Read the model definition and answer for the solid it produces. Units are mm, in the model's axes. A direction names the side the tool comes from. Coordinates: 2 decimals unless noted, no trailing zeros. Loops run counter-clockwise (first coordinate to the right, second up) from the corner with the lowest first, then second, coordinate; pieces in that order, holes last. Notation, with made-up numbers: (20.25, 11.25) - (26.25, 11.25) arc R29 ccw to (26.25, 31.25) - close; hole circle Ø7 at (71.25, 69.25). An arc over 180 degrees is marked (long way). Use one line per item in the form item = value. Start each with the question number.
1) A cutting plane is placed at D-D (z = 6). Give the vertices of the cut face in (x, y).
2) Consider line 1 (X direction, y = 0.25, z = 80); line 2 (Y direction, x = 0, z = -1.2). Determine where each line is inside the solid, lowest interval first.
3) Each of these flat-tipped pins is pushed along its axis until it touches: P1, Ø0.6, axis at x = 7, z = 120, coming from the -Y side; P2, Ø4, axis at x = 3, z = 97.5, coming from the -Y side; P3, Ø4, axis at x = -10, y = -1, coming from the +Z side. Where does it stop, or does it pass through?
4) The mould has two halves that part along X. Classify faces 4 (the face through (5.718, 1.801, -1.002)), 5 (the face through (-7, 7, 120.396)), 6 (the face through (6, -3, 119.888)): released by +X, released by -X, zero draft, split by the parting line, or undercut.
5) A cutting plane is placed at B-B (z = 72.5). Give the vertices of the cut face in (x, y).
6) A cutting plane is placed at A-A (y = 0). Give the vertices of the cut face in (x, z), and give its area (3 significant figures).
7) Which of the six approach directions +Z, -Z, +X, -X, +Y, -Y give full straight-line access (tool end or side, diameter ignored) to faces 1 (the face through (6, -3, 0)), 2 (the face through (-2.808, -12.646, 59.105)), 3 (the face through (0, 0, 71.12))?
from build123d import *

# Parameters (mm, degrees)
F0_R      = 12.954
F0_R_2    = 5.9944
F0_R_3    = 4.0132
F1_DEPTH  = 119.888
F2_R      = 5.9944
F2_R_2    = 4.0132
F3_DEPTH  = 2.032
F5_R      = 5.9944
F5_R_2    = 4.0132
F6_DEPTH  = 2.032
F7_R      = 4.0132
F8_DEPTH  = 50.8
F10_DEPTH = 0.508


# Not quite as in the source:
# - the program builds the solid bodies; features that only make, move or delete a surface that nothing else refers to are left out


with BuildPart() as f1:
    # F0 (on Top) → F1 (new body)
    with BuildSketch(Plane.XY):
        Circle(F0_R)
        Circle(F0_R_2, mode=Mode.SUBTRACT)
        Circle(F0_R_2)
        Circle(F0_R_3, mode=Mode.SUBTRACT)
        Circle(F0_R_3)
    extrude(amount=F1_DEPTH)

    # F2 (on face) → F3 (join)
    with BuildSketch(Plane.XY.offset(119.888)):
        Circle(F2_R)
        Circle(F2_R_2, mode=Mode.SUBTRACT)
    extrude(amount=F3_DEPTH)

    # F5 (on face) + F0 (on Top) → F6 (join)
    with BuildSketch(Plane.XY):
        Circle(F5_R)
        Circle(F5_R_2, mode=Mode.SUBTRACT)
    with BuildSketch(Plane.XY):
        Circle(F0_R_2)
        Circle(F0_R_3, mode=Mode.SUBTRACT)
    extrude(amount=-F6_DEPTH)

    # F7 (on face) → F8 (cut)
    with BuildSketch(Plane.XY.offset(121.92)):
        Circle(F7_R)
    extrude(amount=-F8_DEPTH, mode=Mode.SUBTRACT)

    # F9 (on face) → F10 (join)
    with BuildSketch(Plane.XY.offset(119.888)):
        Polygon((5.5737421783, -7.205022499), (7.205022499, -7.205022499), (7.205022499, -5.7922923006), (6.3893823387, -5.7922923006), align=None)
        Polygon((7.205022499, -5.7922923006), (7.205022499, -7.205022499), (5.5737421783, -7.205022499), (6.3893823387, -8.6177526973), (8.0206626593, -8.6177526973), (8.8363028196, -7.205022499), (8.0206626593, -5.7922923006), align=None)
        Polygon((-6.3893823387, -8.6177526973), (-5.5737421783, -7.205022499), (-7.205022499, -7.205022499), (-7.205022499, -5.7922923006), (-8.0206626593, -5.7922923006), (-8.8363028196, -7.205022499), (-8.0206626593, -8.6177526973), align=None)
        Polygon((-7.205022499, -7.205022499), (-5.5737421783, -7.205022499), (-6.3893823387, -5.7922923006), (-7.205022499, -5.7922923006), align=None)
        Polygon((-7.205022499, 7.205022499), (-7.205022499, 5.6622778066), (-6.3143184355, 5.6622778066), (-5.4236143721, 7.205022499), align=None)
        Polygon((-8.0957265624, 5.6622778066), (-7.205022499, 5.6622778066), (-7.205022499, 7.205022499), (-5.4236143721, 7.205022499), (-6.3143184355, 8.7477671914), (-8.0957265624, 8.7477671914), (-8.9864306259, 7.205022499), align=None)
        Polygon((7.205022499, 7.205022499), (7.205022499, 5.6622778066), (8.0957265624, 5.6622778066), (8.9864306259, 7.205022499), (8.0957265624, 8.7477671914), (6.3143184355, 8.7477671914), (5.4236143721, 7.205022499), align=None)
        Polygon((6.3143184355, 5.6622778066), (7.205022499, 5.6622778066), (7.205022499, 7.205022499), (5.4236143721, 7.205022499), align=None)
    extrude(amount=F10_DEPTH)


solid = f1.part
Found:
q1.outline = circle Ø25.91 at (0, 0)
q2.line_1 = -12.95 to -4.01, 4.01 to 12.95
q2.line_2 = -5.99 to -4.01, 4.01 to 5.99
q3.P1 = -11.07
q3.P2 = -12.92
q3.P3 = 119.89
q4.face_4 = split by the parting line
q4.face_5 = zero draft
q4.face_6 = undercut
q5.outline = circle Ø25.91 at (0, 0); hole circle Ø8.03 at (0, 0)
q6.outline = (-12.95, 0) - (-5.99, 0) - (-5.99, -2.03) - (-4.01, -2.03) - (-4.01, 0) - (4.01, 0) - (4.01, -2.03) - (5.99, -2.03) - (5.99, 0) - (12.95, 0) - (12.95, 119.89) - (5.99, 119.89) - (5.99, 121.92) - (4.01, 121.92) - (4.01, 71.12) - (-4.01, 71.12) - (-4.01, 121.92) - (-5.99, 121.92) - (-5.99, 119.89) - (-12.95, 119.89) - close
q6.area = 2,730 mm^2
q7.face_1 = -Z
q7.face_2 = +Z, -Z
q7.face_3 = +Z
